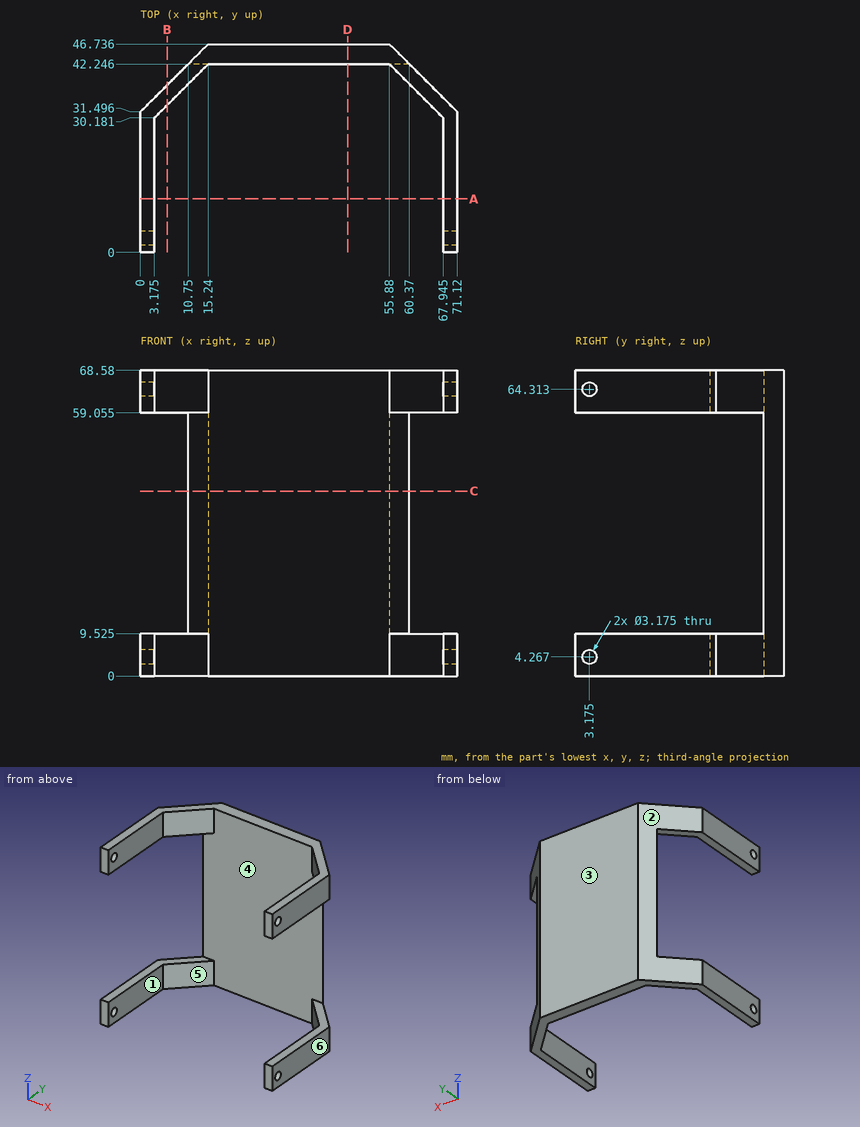
Input: dimensioned drawing with shaded views. Units: mm. Origin: part minimum x, y, z. A direction names the side the tool comes from. Give positions to 0.01 mm unless a question says otherwise; leave off trailing zeros. Write each loop counter-clockwise with the first axis right and the second up, starting at its lowest first coordinate (ties: lowest second). Pieces come first, ordered by that corner, then holes.
1. Section query D-D (x = 46.5). Return the cut outline in (y, z).
2. Section query B-B (x = 6). Return the cut outline in (y, z) (1 decimal).
3. First-contact query: pin 1 (10 mm diameter, centred on y = 8.5, z = 51, fed in from +X). Flat tip, straight axial feed; report the tip coordinate or a pass-through.
4. Material intervals for line 1 along X through (y, z) = (26.5, 60.5) (3 decimals); line 2 along Y through (x, z) = (53.5, 32); line 3 along Y through (x, z) = (13, 14) (1 decimal), sorted ascending.
5. Pull-direction query (X, two-part tool) for the marked faces 1, 2, 3 and 4; classes: +X half, -X half, draft (parallel to the pull), parting line (faces both ways), or undercut.
6. Section query A-A (y = 12). Return the cut outline in (x, z) (3 decimals).
7. Access query for the marked faces 5 and 6. Directions: +Z, -Z, +X, -X, +Y, -Y. A direction counts if a zero-diameter tool reaches every point of the face in a straight line with its end or side. Return the directions, or none.
8. Section query C-C (z = 41.5). Return the cut outline in (x, y).
Output values:
1. outline: (42.25, 0) - (46.74, 0) - (46.74, 68.58) - (42.25, 68.58) - close
2. outline: (33, 0) - (37.5, 0) - (37.5, 9.5) - (33, 9.5) - close; (33, 59.1) - (37.5, 59.1) - (37.5, 68.6) - (33, 68.6) - close
3. pin 1: passes through
4. line 1: x = 0 to 3.175, 67.945 to 71.12
4. line 2: y = 42.25 to 46.74
4. line 3: y = 42.2 to 44.5
5. face 1: undercut
5. face 2: -X half
5. face 3: draft
5. face 4: undercut
6. outline: (0, 0) - (3.175, 0) - (3.175, 9.525) - (0, 9.525) - close; (0, 59.055) - (3.175, 59.055) - (3.175, 68.58) - (0, 68.58) - close; (67.945, 0) - (71.12, 0) - (71.12, 9.525) - (67.945, 9.525) - close; (67.945, 59.055) - (71.12, 59.055) - (71.12, 68.58) - (67.945, 68.58) - close
7. face 5: +Z, -Z, -Y
7. face 6: +Z, -Z, +X, +Y, -Y
8. outline: (10.75, 42.25) - (60.37, 42.25) - (55.88, 46.74) - (15.24, 46.74) - close
